from build123d import *

# Parameters (mm, degrees)
SKETCH2_R           = 8.35
SKETCH4_R           = 8.35
BOSS_EXTRUDE2_DEPTH = 13
BOSS_EXTRUDE3_DEPTH = 13
SKETCH7_R           = 8.35
BOSS_EXTRUDE4_DEPTH = 80
SKETCH8_R           = 8.35
BOSS_EXTRUDE5_DEPTH = 80


with BuildPart() as part:
    # Sweep1: sweep along a path in Sketch1
    with BuildLine(Plane(origin=(0, 0, 0), x_dir=(1, 0, 0), z_dir=(0, 1, 0))) as sweep1_path:
        Line((-300, 0), (-300, -100))
        ThreePointArc((-300, -100), (-288.284271247, -128.284271247), (-260, -140))
        Line((-260, -140), (260, -140))
        ThreePointArc((260, -140), (288.284271247, -128.284271247), (300, -100))
        Line((300, -100), (300, 0))
    # Sketch2 → Sweep1 (sweep)
    with BuildSketch(Plane.XY):
        with Locations((300, 0)):
            Circle(SKETCH2_R)
    sweep(path=sweep1_path.line)

    # Sweep2: sweep along a path in Sketch3
    with BuildLine(Plane.XY.offset(140)) as sweep2_path:
        Line((-252.853261493, -9.077244013), (-246.547005384, -20))
        ThreePointArc((-246.547005384, -20), (-231.905989232, -34.641016151), (-211.905989232, -40))
        Line((-211.905989232, -40), (211.905989232, -40))
        ThreePointArc((211.905989232, -40), (231.905989232, -34.641016151), (246.547005384, -20))
        Line((246.547005384, -20), (252.853261493, -9.077244013))
    # Sketch4 → Sweep2 (sweep)
    with BuildSketch(Plane(origin=(-252.853261493, -9.077244013, 140), x_dir=(0.866025404, 0.5, 0), z_dir=(-0.5, 0.866025404, 0))):
        Circle(SKETCH4_R)
    sweep(path=sweep2_path.line)

    # Sketch5 → Boss-Extrude2 (add)
    with BuildSketch(Plane(origin=(-59.282753417, 102.680740932, 0), x_dir=(0.866025404, 0.5, 0), z_dir=(-0.5, 0.866025404, 0))):
        with BuildLine():
            ThreePointArc((-217.464473881, -134.246575276), (-231.865969889, -140), (-217.464473881, -145.753424724))
            add(Edge.make_bspline(
                [(-217.464473881, -134.246575276), (-228.404544239, -140), (-217.464473881, -145.753424724)],
                knots=[2.381438875, 2.381438875, 2.381438875, 3.901746432, 3.901746432, 3.901746432], degree=2, weights=[1, 0.724730061, 1]))
        make_face()
    extrude(amount=BOSS_EXTRUDE2_DEPTH)

    # Sketch6 → Boss-Extrude3 (add)
    with BuildSketch(Plane(origin=(59.282753417, 102.680740932, 0), x_dir=(0.866025404, -0.5, 0), z_dir=(0.5, 0.866025404, 0))):
        with BuildLine():
            ThreePointArc((217.464473881, -145.753424724), (231.865969889, -140), (217.464473881, -134.246575276))
            add(Edge.make_bspline(
                [(217.464473881, -145.753424724), (228.404544239, -140), (217.464473881, -134.246575276)],
                knots=[5.523031529, 5.523031529, 5.523031529, 7.043339086, 7.043339086, 7.043339086], degree=2, weights=[1, 0.724730061, 1]))
        make_face()
    extrude(amount=BOSS_EXTRUDE3_DEPTH)

    # Sketch7 → Boss-Extrude4 (add)
    with BuildSketch(Plane(origin=(0, 0, 0), x_dir=(-1, 0, 0), z_dir=(0, 0, -1))):
        with Locations((-300, 0)):
            Circle(SKETCH7_R)
    extrude(amount=BOSS_EXTRUDE4_DEPTH)

    # Sketch8 → Boss-Extrude5 (add)
    with BuildSketch(Plane(origin=(0, 0, 0), x_dir=(-1, 0, 0), z_dir=(0, 0, -1))):
        with Locations((300, 0)):
            Circle(SKETCH8_R)
    extrude(amount=BOSS_EXTRUDE5_DEPTH)


solid = part.part
Input: part model. Units: mm. Frame: model coordinates. A direction names the side the tool comes from. Give positions to 0.01 mm unless a question says otherwise; leave off trailing zeros. Write each loop counter-clockwise with the first axis right and the second up, starting at its lowest first coordinate (ties: lowest second). Pieces come first, ordered by that corner, then holes.
Q1. Material intervals for probe 1 along X at (y, z) = (5.5, 74); probe 2 along X at (y, z) = (-20, 134); probe 3 along Z at (x, y) = (-49.5, -7.5), sorted ascending.
Q2. Section A-A, the plane x = -49.5. Output: boundary loops of the cut face in (y, z).
Q3. Set-up query: faces 3 (the face through (2.97, -41.81, 131.85)), 4 (the face through (-300, 0, -80)). Return all of +Z, -Z, +X, -X, +Y, -Y with unobstructed straight access to the full face (end or side cutting, diameter ignored); none if empty.
Q4. Pull-direction query (Y, two-part tool) for faces 1 (the face through (3.64, -5.643, 133.846)), 2 (the face through (300, 0, -80)); classes: pulls with the +Y half, pulls with the -Y half, needs draft (parallel to the pull), parting line crosses it, or undercut.
Q5. First-contact query: P1, Ø1.5, axis at x = -83, y = -6.5, coming from the -Z side; P2, Ø1.5, axis at y = -6, z = 98, coming from the -X side. Flat tips, straight axial feed; report the tip coordinate or a pass-through.
Q6. Section B-B, the plane z = 92.5. Output: boundary loops of the cut face in (x, y), plus the area to 3 significant figures.
Filled in:
1. probe 1: x = -306.28 to -293.72, 293.72 to 306.28
1. probe 2: x = -253.25 to -239.64, 239.64 to 253.25
1. probe 3: z = 136.33 to 143.67
2. outline: circle Ø16.7 at (-40, 140); circle Ø16.7 at (0, 140)
3. face 3: none
3. face 4: -Z, +X, -X, +Y, -Y
4. face 1: undercut
4. face 2: needs draft
5. P1: stops at z = 133.95
5. P2: stops at x = -306.49
6. outline: circle Ø16.7 at (-300, 0); circle Ø16.7 at (300, 0)
6. area: 438 mm2
